Read the model definition and answer for the solid it produces. Units are mm, in the model's axes. Face numbers are marked on the shaded views. Coordinates: 2 decimals unless noted, no trailing zeros. Write each loop counter-clockwise with the first axis right and the second up, starting at its lowest first coordinate (ties: lowest second). Pieces come first, ordered by that corner, then holes.
1) Each of these flat-tipped pins is pushed along its axis until it touches: pin 1 Ø3 at (x, z) = (-30.5, 17.5) entering from +Y; pin 2 Ø8 at (y, z) = (-7, 15.5) entering from +X; pin 3 Ø3 at (x, z) = (12.5, 19) entering from -Y. Where does it stop, or does it pass through?
2) The part is cut by section C-C (y = -15.5). Determine the outline of the cut face in (x, z).
3) Find the intervals of material crossed by line 1 (X direction, y = -11, z = 18.25); line 2 (X direction, y = -1, z = 10); line 3 (Y direction, x = -28, z = 9.75), in increasing order.
4) Determine the mould class of the marked faces 1 and 2 for opening direction X: +X half, -X half, draft (parallel to the pull), parting line (faces both ways), or undercut.
5) The part is cut by section A-A (z = 9.25). Determine the outline of the cut face in (x, y).
6) The part is cut by section B-B (x = -11). Determine the outline of the cut face in (y, z), then the cut area to 3 significant figures.
from build123d import *

# Parameters (mm, degrees)
F2_DEPTH = 25.4


# Not quite as in the source:
# - the program builds the solid bodies; features that only make, move or delete a surface that nothing else refers to are left out


with BuildPart() as f2:
    # F0 (on Top) → F2 (new body)
    with BuildSketch(Plane.XY):
        with BuildLine():
            Line((0, -22.3464633732), (0, 0))
            Line((0, 0), (0, 22.3464633732))
            ThreePointArc((0, 22.3464633732), (-13.4819478567, 17.8213778165), (-21.5037952489, 6.0787511204))
            ThreePointArc((-21.5037952489, 6.0787511204), (-22.3364486511, -0.6689446499), (-21.1014820814, -7.354718163))
            ThreePointArc((-21.1014820814, -7.354718163), (-12.9424202767, -18.216975124), (0, -22.3464633732))
        make_face()
        with BuildLine():
            Line((0, 22.3464633732), (0, 0))
            Line((0, 0), (0, -22.3464633732))
            ThreePointArc((0, -22.3464633732), (15.8013357867, -15.8013357867), (22.3464633732, 0))
            ThreePointArc((22.3464633732, 0), (15.8013357867, 15.8013357867), (0, 22.3464633732))
        make_face()
        with BuildLine():
            ThreePointArc((-21.1014820814, -7.354718163), (-22.3364486511, -0.6689446499), (-21.5037952489, 6.0787511204))
            ThreePointArc((-21.5037952489, 6.0787511204), (-37.8621842038, 7.8047564636), (-52.3418858647, 0))
            ThreePointArc((-52.3418858647, 0), (-37.9892096461, -9.0613878034), (-21.1014820814, -7.354718163))
        make_face()
    extrude(amount=F2_DEPTH)


solid = f2.part
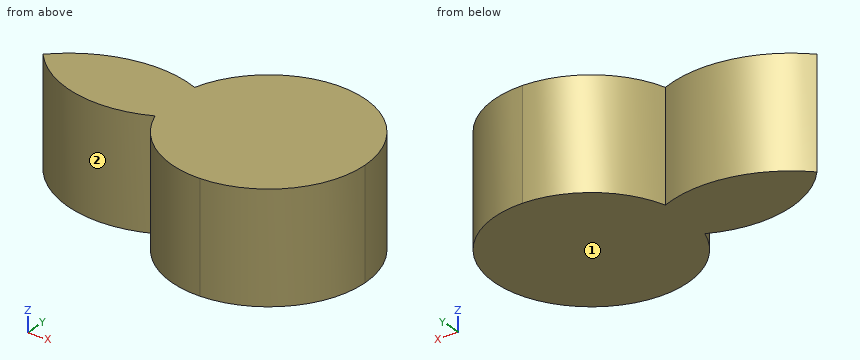
Reported:
1. pin 1: stops at y = 8.33
1. pin 2: stops at x = 22.14
1. pin 3: stops at y = -19.45
2. outline: (-16.1, 0) - (16.1, 0) - (16.1, 25.4) - (-16.1, 25.4) - close
3. line 1: x = -19.45 to 19.45
3. line 2: x = -51.5 to 22.32
3. line 3: y = -9.44 to 7.97
4. face 1: draft
4. face 2: undercut
5. outline: (-52.34, 0) arc R26.04 ccw to (-21.1, -7.35) arc R22.35 ccw (long way) to (-21.5, 6.08) arc R27.85 ccw to start
6. outline: (-19.45, 0) - (19.45, 0) - (19.45, 25.4) - (-19.45, 25.4) - close
6. area: 988 mm2
